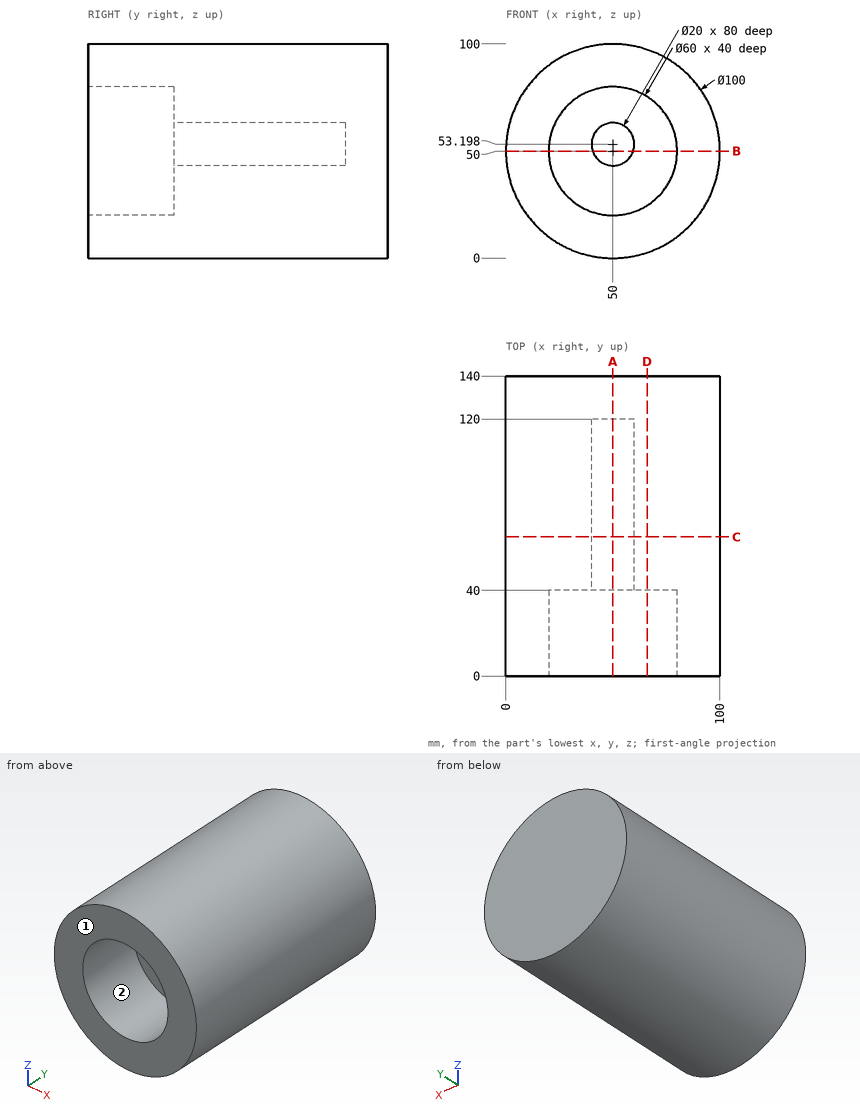
Geometry: see drawing. Coordinates: mm, zero at the bounding-box minimum. A direction names the side the tool comes from. Give positions to 0.01 mm unless a question says otherwise; leave off trailing zeros. Loops run counter-clockwise (first coordinate to the right, second up) from the corner with the lowest first, then second, coordinate; pieces in that order, holes last. Notation, with made-up numbers: (11.25, 64.5) - (21.25, 64.5) arc R27 ccw to (21.25, 99.5) - close; hole circle Ø7 at (87, 23.5). An arc over 180 degrees is marked (long way). Use CSV: the item, a comma, the result in double quotes. Start each with the question number.
Item 1: Section A-A on x = 50. Return loops of the section in (y, z).
Item 2: Section C-C on y = 65. Return loops of the section in (x, z), then the cut area to 3 significant figures.
Item 3: Contact query for flat-ended pins moving along their axis: P1, Ø4, axis at x = 69, z = 30.5, coming from the -Y side; P2, Ø5, axis at x = 42, y = 28, coming from the -Z side; P3, Ø6, axis at y = 122, z = 31.5, coming from the -X side; P4, Ø1.5, axis at x = 49.5, z = 15.5, coming from the -Y side. Output: stop coordinate, or through.
Item 4: Line query: line 1 (Z direction, x = 50, y = 24.5); line 2 (Z direction, x = 50, y = 82.5); line 3 (Y direction, x = 32, z = 55.5). Output: solid intervals per line, ascending.
Item 5: Reachability of the marked faces 1 and 2 from +Z, -Z, +X, -X, +Y, -Y: full face, straight path, thin tool, end or side. Return the list, or none.
Item 6: Section B-B on z = 50. Return loops of the section in (x, y) (3 decimals).
Item 7: Section D-D on x = 66. Return loops of the section in (y, z), then the cut area to 3 significant figures.
Ans:
1,outline,"(0, 0) - (140, 0) - (140, 100) - (0, 100) - (0, 80) - (40, 80) - (40, 63.2) - (120, 63.2) - (120, 43.2) - (40, 43.2) - (40, 20) - (0, 20) - close"
2,outline,"circle Ø100 at (50, 50); hole circle Ø20 at (50, 53.2)"
2,area,"7,540 mm2"
3,P1,"stops at y = 40"
3,P2,"stops at z = 0.3"
3,P3,"stops at x = 2.46"
3,P4,"stops at y = 0"
4,line 1,"z = 0 to 20, 80 to 100"
4,line 2,"z = 0 to 43.2, 63.2 to 100"
4,line 3,"y = 40 to 140"
5,face 1,"+Z, -Z, +X, -X, -Y"
5,face 2,"-Y"
6,outline,"(0, 0) - (20, 0) - (20, 40) - (40.525, 40) - (40.525, 120) - (59.475, 120) - (59.475, 40) - (80, 40) - (80, 0) - (100, 0) - (100, 140) - (0, 140) - close"
7,outline,"(0, 2.63) - (140, 2.63) - (140, 97.37) - (0, 97.37) - (0, 75.38) - (40, 75.38) - (40, 24.62) - (0, 24.62) - close"
7,area,"11,200 mm2"
